```python
from build123d import *

# Parameters (mm, degrees)
SKETCH1_R               = 10
BOSS_EXTRUDE1_DEPTH     = 8
SKETCH2_R               = 13.5
CUT_EXTRUDE1_DEPTH      = 2
SKETCH3_R               = 13.5
CUT_EXTRUDE2_DEPTH      = 2
CUT_EXTRUDE3_DEPTH      = 15.696938457
CUT_EXTRUDE3_DEPTH_BACK = 15.696938457
SKETCH4_R               = 2.25


with BuildPart() as part:
    # Sketch1 → Boss-Extrude1 (new body)
    with BuildSketch(Plane(origin=(0, 0, 0), x_dir=(0, 0, -1), z_dir=(1, 0, 0))):
        Circle(SKETCH1_R)
    extrude(amount=BOSS_EXTRUDE1_DEPTH)

    # Sketch2 → Cut-Extrude1 (cut)
    with BuildSketch(Plane(origin=(8, 0, 0), x_dir=(0, 0, -1), z_dir=(1, 0, 0))):
        Circle(SKETCH2_R)
    extrude(amount=-CUT_EXTRUDE1_DEPTH, mode=Mode.SUBTRACT)

    # Sketch3 → Cut-Extrude2 (cut)
    with BuildSketch(Plane.ZY):
        Circle(SKETCH3_R)
    extrude(amount=-CUT_EXTRUDE2_DEPTH, mode=Mode.SUBTRACT)

    # Sketch4 → Cut-Extrude3 (cut, two sides: drawn at the far end of the back side and taken through both)
    with BuildSketch(Plane.ZY.offset(-2).offset(-CUT_EXTRUDE3_DEPTH_BACK)):
        Circle(SKETCH4_R)
    extrude(amount=CUT_EXTRUDE3_DEPTH + CUT_EXTRUDE3_DEPTH_BACK, mode=Mode.SUBTRACT)


solid = part.part
```
Work out the finished part from the listing and answer in its coordinate system (mm). Round coordinates to 2 decimals unless told otherwise and drop trailing zeros. Write each loop counter-clockwise with the first axis right and the second up, starting at its lowest first coordinate (ties: lowest second). Pieces come first, ordered by that corner, then holes. Notation, with made-up numbers: (53.5, 22.25) - (90.5, 22.25) arc R32 ccw to (90.5, 57.25) - close; hole circle Ø6 at (15.25, 16). An arc over 180 degrees is marked (long way). Return JSON: item names as keys, results as strings. Group by question number.
Q1. The part is cut by section B-B on x = 4.5. Write down the section's boundary in (y, z), then the cut area to 3 significant figures.
Q2. The part is cut by section D-D on z = 7. Write down the section's boundary in (x, y), then the cut area to 3 significant figures.
Q3. Each of these flat-tipped pins is pushed along its axis until it touches: pin 1 Ø1.5 at (x, z) = (5, -5.5) entering from +Y; pin 2 Ø1 at (x, z) = (4.5, -3) entering from -Y; pin 3 Ø1.5 at (x, z) = (2.5, -6) entering from +Y; pin 4 Ø2.5 at (y, z) = (0, 0) entering from -X. Where does it stop, or does it pass through?
Q4. The part is cut by section A-A on y = 0. Write down the section's boundary in (x, z).
Q5. The mould has two halves that part along Z. Classify faces 1 (the cylindrical face through (4.03, 2.23, -0.29)), 2 (the flat face through (2, 2.4, -0.1)), 3 (the cylindrical face through (3.97, -9.76, 2.17)): released by +Z, released by -Z, zero draft, split by the parting line, or undercut.
Q6. Find the intervals of material crossed by L1, parallel to Z at x = 3.95, y = 0; L2, parallel to Z at x = 3.5, y = -1.75, in increasing order.
Q7. The part is cut by section C-C on y = 8. Write down the section's boundary in (x, z).
Solved:
{
 "1": {"outline": "circle Ø20 at (0, 0); hole circle Ø4.5 at (0, 0)", "area": "298 mm²"},
 "2": {"outline": "(2, -7.14) - (6, -7.14) - (6, 7.14) - (2, 7.14) - close", "area": "57.1 mm²"},
 "3": {"pin 1": "y = 8.8", "pin 2": "y = -9.68", "pin 3": "y = 8.51", "pin 4": "through"},
 "4": {"outline": "(2, -10) - (6, -10) - (6, -2.25) - (2, -2.25) - close; (2, 2.25) - (6, 2.25) - (6, 10) - (2, 10) - close"},
 "5": {"face 1": "undercut", "face 2": "zero draft", "face 3": "split by the parting line"},
 "6": {"L1": "-10 to -2.25, 2.25 to 10", "L2": "-9.85 to -1.41, 1.41 to 9.85"},
 "7": {"outline": "(2, -6) - (6, -6) - (6, 6) - (2, 6) - close"}
}
